from build123d import *

# Parameters (mm, degrees)
BOSS_EXTRUDE1_DEPTH = 7.5
FILLET1_R           = 10
SKETCH2_R           = 4.975
CUT_EXTRUDE1_DEPTH  = 5
CHAMFER2_SIZE       = 1.5


with BuildPart() as part:
    # Sketch1 → Boss-Extrude1 (new body)
    with BuildSketch(Plane(origin=(0, 0, 0), x_dir=(1, 0, 0), z_dir=(0, 1, 0))):
        Polygon((80, 0), (20, 0), (20, -20), (0, -20), (0, -80), (20, -80), (20, -100), (80, -100), (80, -80), (100, -80), (100, -20), (80, -20), align=None)
    extrude(amount=BOSS_EXTRUDE1_DEPTH)

    # Fillet1
    # the kernel refuses this fillet: 10 mm, written as the material it takes off along each edge
    with BuildSketch(Plane(origin=(-24.206145914, 7.5, 80), x_dir=(0, -1, 0), z_dir=(1, 0, 0)), Plane(origin=(20, 7.5, 80), x_dir=(0, -1, 0), z_dir=(0, 0, 1)), Plane(origin=(80, 7.5, 124.206145914), x_dir=(0, -1, 0), z_dir=(0, 0, -1)), Plane(origin=(80, 7.5, 80), x_dir=(0, -1, 0), z_dir=(1, 0, 0)), Plane(origin=(124.206145914, 7.5, 20), x_dir=(0, -1, 0), z_dir=(-1, 0, 0)), Plane(origin=(80, 7.5, 20), x_dir=(0, -1, 0), z_dir=(0, 0, -1)), Plane(origin=(20, 7.5, -24.206145914), x_dir=(0, -1, 0), z_dir=(0, 0, 1)), Plane(origin=(20, 7.5, 20), x_dir=(0, -1, 0), z_dir=(-1, 0, 0))) as fillet1_piece_1:
        with BuildLine():
            CenterArc((10, 9.682458366), FILLET1_R, 180, 75.522487814)
            Line((0, 9.682458366), (-0.2, 9.682458366))
            Line((-0.2, 9.682458366), (-0.2, 0))
            Line((-0.2, 0), (0, -0.2))
            ThreePointArc((0, -0.2), (3.75, -0.2), (7.45, -0.193649167))
            Line((7.45, -0.193649167), (7.5, 0))
        make_face()
    extrude(amount=44.206145914, mode=Mode.SUBTRACT)
    with BuildSketch(Plane(origin=(-4.206145914, 7.5, 100), x_dir=(0, -1, 0), z_dir=(1, 0, 0)), Plane(origin=(100, 7.5, 104.206145914), x_dir=(0, -1, 0), z_dir=(0, 0, -1)), Plane(origin=(104.206145914, 7.5, 0), x_dir=(0, -1, 0), z_dir=(-1, 0, 0)), Plane(origin=(0, 7.5, -4.206145914), x_dir=(0, -1, 0), z_dir=(0, 0, 1))) as fillet1_piece_2:
        with BuildLine():
            CenterArc((10, 9.682458366), FILLET1_R, 180, 75.522487814)
            Line((0, 9.682458366), (-0.2, 9.682458366))
            Line((-0.2, 9.682458366), (-0.2, 0))
            Line((-0.2, 0), (0, -0.2))
            ThreePointArc((0, -0.2), (3.75, -0.2), (7.45, -0.193649167))
            Line((7.45, -0.193649167), (7.5, 0))
        make_face()
    extrude(amount=108.412291828, mode=Mode.SUBTRACT)
    with BuildSketch(Plane(origin=(-24.206145914, 7.5, 80), x_dir=(0, -1, 0), z_dir=(1, 0, 0))) as fillet1_piece_3a_section:
        with BuildLine():
            CenterArc((10, 9.682458366), FILLET1_R, 180, 75.522487814)
            Line((0, 9.682458366), (-0.2, 9.682458366))
            Line((-0.2, 9.682458366), (-0.2, 0))
            Line((-0.2, 0), (0, -0.2))
            ThreePointArc((0, -0.2), (3.75, -0.2), (7.45, -0.193649167))
            Line((7.45, -0.193649167), (7.5, 0))
        make_face()
    fillet1_piece_3a = extrude(amount=68.412291828, mode=Mode.PRIVATE)
    fillet1_piece_3a = split(fillet1_piece_3a, bisect_by=Plane(origin=(20, 5.604082443, 77.718558992), z_dir=(1, 0, 0)), keep=Keep.TOP, mode=Mode.PRIVATE)
    with BuildSketch(Plane(origin=(20, 7.5, 55.793854086), x_dir=(0, -1, 0), z_dir=(0, 0, 1))) as fillet1_piece_3b_section:
        with BuildLine():
            CenterArc((10, 9.682458366), FILLET1_R, 180, 75.522487814)
            Line((0, 9.682458366), (-0.2, 9.682458366))
            Line((-0.2, 9.682458366), (-0.2, 0))
            Line((-0.2, 0), (0, -0.2))
            ThreePointArc((0, -0.2), (3.75, -0.2), (7.45, -0.193649167))
            Line((7.45, -0.193649167), (7.5, 0))
        make_face()
    fillet1_piece_3b = extrude(amount=68.412291828, mode=Mode.PRIVATE)
    fillet1_piece_3b = split(fillet1_piece_3b, bisect_by=Plane(origin=(22.281441008, 5.604082443, 80), z_dir=(0, 0, -1)), keep=Keep.TOP, mode=Mode.PRIVATE)
    fillet1_piece_3 = fillet1_piece_3a & fillet1_piece_3b
    add(fillet1_piece_3, mode=Mode.SUBTRACT)
    with BuildSketch(Plane(origin=(80, 7.5, 124.206145914), x_dir=(0, -1, 0), z_dir=(0, 0, -1))) as fillet1_piece_4a_section:
        with BuildLine():
            CenterArc((10, 9.682458366), FILLET1_R, 180, 75.522487814)
            Line((0, 9.682458366), (-0.2, 9.682458366))
            Line((-0.2, 9.682458366), (-0.2, 0))
            Line((-0.2, 0), (0, -0.2))
            ThreePointArc((0, -0.2), (3.75, -0.2), (7.45, -0.193649167))
            Line((7.45, -0.193649167), (7.5, 0))
        make_face()
    fillet1_piece_4a = extrude(amount=68.412291828, mode=Mode.PRIVATE)
    fillet1_piece_4a = split(fillet1_piece_4a, bisect_by=Plane(origin=(77.718558992, 5.604082443, 80), z_dir=(0, 0, -1)), keep=Keep.TOP, mode=Mode.PRIVATE)
    with BuildSketch(Plane(origin=(55.793854086, 7.5, 80), x_dir=(0, -1, 0), z_dir=(1, 0, 0))) as fillet1_piece_4b_section:
        with BuildLine():
            CenterArc((10, 9.682458366), FILLET1_R, 180, 75.522487814)
            Line((0, 9.682458366), (-0.2, 9.682458366))
            Line((-0.2, 9.682458366), (-0.2, 0))
            Line((-0.2, 0), (0, -0.2))
            ThreePointArc((0, -0.2), (3.75, -0.2), (7.45, -0.193649167))
            Line((7.45, -0.193649167), (7.5, 0))
        make_face()
    fillet1_piece_4b = extrude(amount=68.412291828, mode=Mode.PRIVATE)
    fillet1_piece_4b = split(fillet1_piece_4b, bisect_by=Plane(origin=(80, 5.604082443, 77.718558992), z_dir=(-1, 0, 0)), keep=Keep.TOP, mode=Mode.PRIVATE)
    fillet1_piece_4 = fillet1_piece_4a & fillet1_piece_4b
    add(fillet1_piece_4, mode=Mode.SUBTRACT)
    with BuildSketch(Plane(origin=(124.206145914, 7.5, 20), x_dir=(0, -1, 0), z_dir=(-1, 0, 0))) as fillet1_piece_5a_section:
        with BuildLine():
            CenterArc((10, 9.682458366), FILLET1_R, 180, 75.522487814)
            Line((0, 9.682458366), (-0.2, 9.682458366))
            Line((-0.2, 9.682458366), (-0.2, 0))
            Line((-0.2, 0), (0, -0.2))
            ThreePointArc((0, -0.2), (3.75, -0.2), (7.45, -0.193649167))
            Line((7.45, -0.193649167), (7.5, 0))
        make_face()
    fillet1_piece_5a = extrude(amount=68.412291828, mode=Mode.PRIVATE)
    fillet1_piece_5a = split(fillet1_piece_5a, bisect_by=Plane(origin=(80, 5.604082443, 22.281441008), z_dir=(-1, 0, 0)), keep=Keep.TOP, mode=Mode.PRIVATE)
    with BuildSketch(Plane(origin=(80, 7.5, 44.206145914), x_dir=(0, -1, 0), z_dir=(0, 0, -1))) as fillet1_piece_5b_section:
        with BuildLine():
            CenterArc((10, 9.682458366), FILLET1_R, 180, 75.522487814)
            Line((0, 9.682458366), (-0.2, 9.682458366))
            Line((-0.2, 9.682458366), (-0.2, 0))
            Line((-0.2, 0), (0, -0.2))
            ThreePointArc((0, -0.2), (3.75, -0.2), (7.45, -0.193649167))
            Line((7.45, -0.193649167), (7.5, 0))
        make_face()
    fillet1_piece_5b = extrude(amount=68.412291828, mode=Mode.PRIVATE)
    fillet1_piece_5b = split(fillet1_piece_5b, bisect_by=Plane(origin=(77.718558992, 5.604082443, 20), z_dir=(0, 0, 1)), keep=Keep.TOP, mode=Mode.PRIVATE)
    fillet1_piece_5 = fillet1_piece_5a & fillet1_piece_5b
    add(fillet1_piece_5, mode=Mode.SUBTRACT)
    with BuildSketch(Plane(origin=(20, 7.5, -24.206145914), x_dir=(0, -1, 0), z_dir=(0, 0, 1))) as fillet1_piece_6a_section:
        with BuildLine():
            CenterArc((10, 9.682458366), FILLET1_R, 180, 75.522487814)
            Line((0, 9.682458366), (-0.2, 9.682458366))
            Line((-0.2, 9.682458366), (-0.2, 0))
            Line((-0.2, 0), (0, -0.2))
            ThreePointArc((0, -0.2), (3.75, -0.2), (7.45, -0.193649167))
            Line((7.45, -0.193649167), (7.5, 0))
        make_face()
    fillet1_piece_6a = extrude(amount=68.412291828, mode=Mode.PRIVATE)
    fillet1_piece_6a = split(fillet1_piece_6a, bisect_by=Plane(origin=(22.281441008, 5.604082443, 20), z_dir=(0, 0, 1)), keep=Keep.TOP, mode=Mode.PRIVATE)
    with BuildSketch(Plane(origin=(44.206145914, 7.5, 20), x_dir=(0, -1, 0), z_dir=(-1, 0, 0))) as fillet1_piece_6b_section:
        with BuildLine():
            CenterArc((10, 9.682458366), FILLET1_R, 180, 75.522487814)
            Line((0, 9.682458366), (-0.2, 9.682458366))
            Line((-0.2, 9.682458366), (-0.2, 0))
            Line((-0.2, 0), (0, -0.2))
            ThreePointArc((0, -0.2), (3.75, -0.2), (7.45, -0.193649167))
            Line((7.45, -0.193649167), (7.5, 0))
        make_face()
    fillet1_piece_6b = extrude(amount=68.412291828, mode=Mode.PRIVATE)
    fillet1_piece_6b = split(fillet1_piece_6b, bisect_by=Plane(origin=(20, 5.604082443, 22.281441008), z_dir=(1, 0, 0)), keep=Keep.TOP, mode=Mode.PRIVATE)
    fillet1_piece_6 = fillet1_piece_6a & fillet1_piece_6b
    add(fillet1_piece_6, mode=Mode.SUBTRACT)

    # Sketch2 → Cut-Extrude1 (cut)
    with BuildSketch(Plane(origin=(0, 7.5, 0), x_dir=(1, 0, 0), z_dir=(0, 1, 0))):
        with Locations(Location((50.317541634, -49.682458366, 0), (0, 0, 270))):
            Circle(SKETCH2_R)
    extrude(amount=-CUT_EXTRUDE1_DEPTH, mode=Mode.SUBTRACT)

    # Chamfer2
    chamfer2_edges = [part.edges().sort_by_distance(p)[0] for p in [
        (50.317541634, 7.5, 44.707458366),
    ]]
    chamfer(chamfer2_edges, length=CHAMFER2_SIZE)


solid = part.part
Build history of the part. All positions in model axes, mm. A direction names the side the tool comes from. Round coordinates to 2 decimals unless told otherwise and drop trailing zeros. Write each loop counter-clockwise with the first axis right and the second up, starting at its lowest first coordinate (ties: lowest second). Pieces come first, ordered by that corner, then holes. Notation, with made-up numbers: M -32.5,69.5 L 3.5,69.5 A25 ccw 3.5,101.5 Z; hole C -30.5,-24 d4. An arc over 180 degrees is marked long. Answer in a Markdown table with one row per item.
1. Mould opens along X. For faces 6 (the face through (47.29, 4.274, 45.734)), 7 (the face through (49.58, 5.46, 96.37)), 8 (the face through (96.37, 5.46, 50.42)) say: +X half, -X half, draft (parallel to the pull), parting line (faces both ways), or undercut.
Geometry check:
| item | result |
|---|---|
| face 6 | undercut |
| face 7 | draft |
| face 8 | +X half |
2. Saw through at C-C (z = 12). List the corners of the cut face in (x, y).
Geometry check:
| item | result |
|---|---|
| outline | M 20,0 L 80,0 A10 ccw 70.32,7.5 L 29.68,7.5 A10 ccw Z |
3. Saw through at D-D (x = 84). List the corners of the cut face in (y, z).
Geometry check:
| item | result |
|---|---|
| outline | M 0,20 A10 ccw 7.5,29.68 L 7.5,70.32 A10 ccw 0,80 Z |
4. Flat gauge pins, fed straight in: P1, Ø2, axis at y = 4.5, z = 56.5, coming from the +X side; P2, Ø1.5, axis at y = 5.5, z = 41.5, coming from the -X side; P3, Ø2, axis at x = 77, y = 4, coming from the -Z side. Where does each tip first touch, or does it go through?
Geometry check:
| item | result |
|---|---|
| P1 | x = 98.32 |
| P2 | x = 2.79 |
| P3 | z = 1.33 |
5. Which spindle directions (+Z, -Z, +X, -X, +Y, -Y) get a long thin tool onto all of the face, cutting with end or side? Do faces 1 (the face through (50, 2.5, 50)), 2 (the face through (23.63, 5.46, 84.95)), 3 (the face through (76.37, 5.46, 85.37)), 4 (the face through (15.05, 5.46, 23.63)), 5 (the face through (76.37, 5.46, 15.05)). Say none if no direction does.
Geometry check:
| item | result |
|---|---|
| face 1 | +Y |
| face 2 | +Z, -X, +Y |
| face 3 | +Z, +X, +Y |
| face 4 | -Z, -X, +Y |
| face 5 | -Z, +X, +Y |
6. Saw through at A-A (y = 4.5). List the corners of the cut face in (x, z) (3 decimals).
Geometry check:
| item | result |
|---|---|
| outline | M 2.541,22.541 L 22.541,22.541 L 22.541,2.541 L 77.459,2.541 L 77.459,22.541 L 97.459,22.541 L 97.459,77.459 L 77.459,77.459 L 77.459,97.459 L 22.541,97.459 L 22.541,77.459 L 2.541,77.459 Z; hole C 50.318,49.682 d9.95 |
7. Saw through at B-B (x = 27.5). List the corners of the cut face in (y, z).
Geometry check:
| item | result |
|---|---|
| outline | M 0,0 A10 ccw 7.26,7.5 L 7.26,27.5 A10 ccw 7.5,29.68 L 7.5,70.32 A10 ccw 7.26,72.5 L 7.26,92.5 A10 ccw 0,100 Z |
8. Probe L1, parallel to X at y = 5, z = 50; L2, parallel to Y at x = 71, z = 79.5; L3, parallel to X at y = 1, z = 9. List the from-to ranges inside material, lowest first. Write a range as [from, to].
Geometry check:
| item | result |
|---|---|
| L1 | [3.07, 45.35], [55.28, 96.93] |
| L2 | [0, 7.48] |
| L3 | [20.31, 79.69] |
